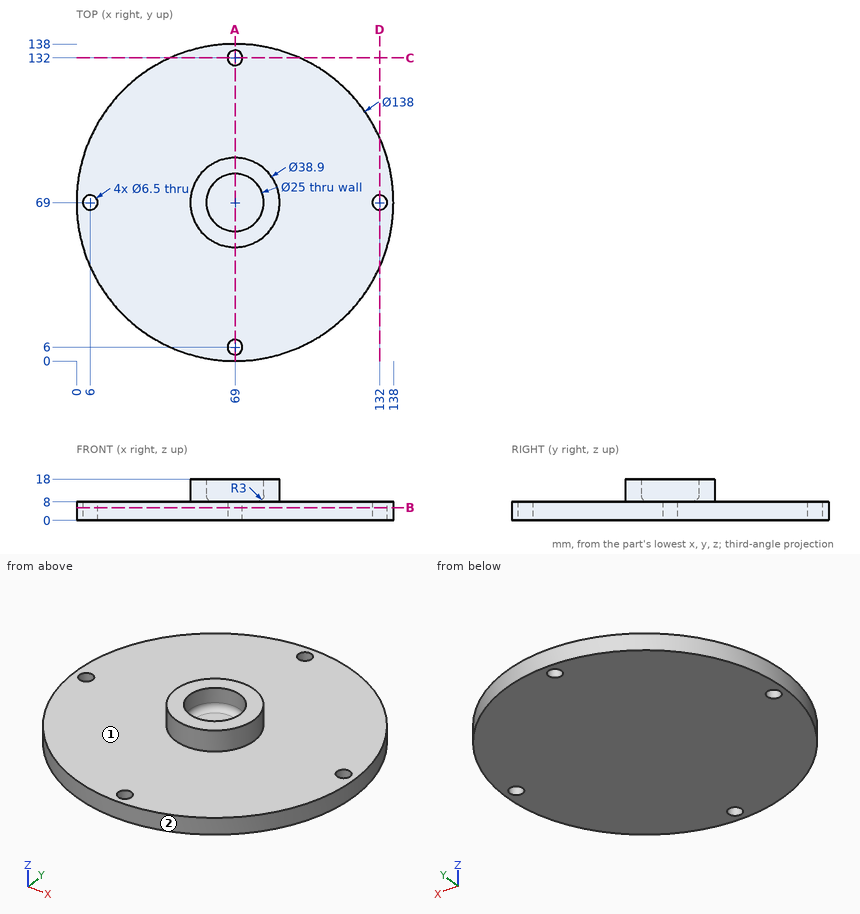
Geometry: see drawing. Coordinates: mm, zero at the bounding-box minimum. A direction names the side the tool comes from. Give positions to 0.01 mm unless a question says otherwise; leave off trailing zeros. Loops run counter-clockwise (first coordinate to the right, second up) from the corner with the lowest first, then second, coordinate; pieces in that order, holes last. Notation, with made-up numbers: (43.25, 57) -> (81.25, 57) arc R10 cw to (81.25, 73) -> close; hole circle Ø9 at (23, -39.5). An arc over 180 degrees is marked (long way). Use one line per item in the form item = value.
Item 1: Section query B-B on z = 5.5. Output: boundary loops of the cut face in (x, y).
A:
outline = circle Ø138 at (69, 69); hole circle Ø6.5 at (6, 69); hole circle Ø6.5 at (69, 6); hole circle Ø6.5 at (69, 132); hole circle Ø6.5 at (132, 69)
Item 2: Line query: probe 1 along Y at (x, z) = (69, 4); probe 2 along Y at (x, z) = (69, 16.25); probe 3 along Z at (x, y) = (50, 97). Output: solid intervals per line, ascending.
A:
probe_1 = 0 to 2.75, 9.25 to 128.75, 135.25 to 138
probe_2 = 49.55 to 56.5, 81.5 to 88.45
probe_3 = 0 to 8
Item 3: Section query C-C on y = 132. Output: boundary loops of the cut face in (x, z), and give its area (3 significant figures).
A:
outline = (40.86, 0) -> (65.75, 0) -> (65.75, 8) -> (40.86, 8) -> close; (72.25, 0) -> (97.14, 0) -> (97.14, 8) -> (72.25, 8) -> close
area = 398 mm^2
Item 4: Pin query (flat end, axial travel): P1, Ø1.5, axis at y = 101.5, z = 2.5, coming from the +X side; P2, Ø6, axis at x = 19.5, z = 8.5, coming from the +Y side; P3, Ø8.5, axis at x = 132, y = 69, coming from the -Z side; P4, Ø22.5, axis at x = 69, y = 69, coming from the +Z side. Return the tip coordinate at first contact, or that it passes through.
A:
P1 = 130.26
P2 = 119.94
P3 = 0
P4 = 8.56
Item 5: Section query A-A on x = 69. Output: boundary loops of the cut face in (y, z).
A:
outline = (0, 0) -> (2.75, 0) -> (2.75, 8) -> (0, 8) -> close; (9.25, 0) -> (128.75, 0) -> (128.75, 8) -> (88.45, 8) -> (88.45, 18) -> (81.5, 18) -> (81.5, 11) arc R3 cw to (78.5, 8) -> (59.5, 8) arc R3 cw to (56.5, 11) -> (56.5, 18) -> (49.55, 18) -> (49.55, 8) -> (9.25, 8) -> close; (135.25, 0) -> (138, 0) -> (138, 8) -> (135.25, 8) -> close
Item 6: Access query for the marked faces 1 and 2. Directions: +Z, -Z, +X, -X, +Y, -Y. A direction counts if a zero-diameter tool reaches every point of the face in a straight line with its end or side. Return the directions, or none.
A:
face_1 = +Z
face_2 = +Z, -Z
